Build history of the part. All positions in model axes, mm. A direction names the side the tool comes from. Give positions to 0.01 mm unless a question says otherwise; leave off trailing zeros. Write each loop counter-clockwise with the first axis right and the second up, starting at its lowest first coordinate (ties: lowest second). Pieces come first, ordered by that corner, then holes. Notation, with made-up numbers: M -13,36 L 33,36 A7 cw 33,40 Z; hole C 2,86.25 d11. An arc over 180 degrees is marked long. One line per item, written item: value. Start each with the question number.
from build123d import *

# Parameters (mm, degrees)
SKETCH1_W           = 254
SKETCH1_H           = 46.99
BOSS_EXTRUDE1_DEPTH = 3.0988
FILLET1_R           = 6.35
SKETCH2_W           = 63.5
SKETCH2_H           = 5.715
CUT_EXTRUDE1_DEPTH  = 130.192173085
SKETCH3_W           = 38.1
SKETCH3_H           = 5.08
CUT_EXTRUDE2_DEPTH  = 130.192173085
CUT_EXTRUDE3_DEPTH  = 130.192173085
FILLET2_R           = 6.35


with BuildPart() as part:
    # Sketch1 → Boss-Extrude1 (new body)
    with BuildSketch(Plane.XY):
        Rectangle(SKETCH1_W, SKETCH1_H)
    extrude(amount=BOSS_EXTRUDE1_DEPTH)

    # Fillet1
    fillet1_edges = [part.edges().sort_by_distance(p)[0] for p in [
        (-127, 23.495, 1.5494),
        (127, 23.495, 1.5494),
    ]]
    fillet(fillet1_edges, radius=FILLET1_R)

    # Sketch2 → Cut-Extrude1 (cut, through all)
    with BuildSketch(Plane.XY.offset(3.0988)):
        with Locations((-95.25, -20.6375)):
            Rectangle(SKETCH2_W, SKETCH2_H)
        with Locations((95.25, -20.6375)):
            Rectangle(SKETCH2_W, SKETCH2_H)
    extrude(amount=-CUT_EXTRUDE1_DEPTH, mode=Mode.SUBTRACT)

    # Sketch3 → Cut-Extrude2 (cut, through all)
    with BuildSketch(Plane.XY.offset(3.0988)):
        with Locations((-102.87, -15.24)):
            Rectangle(SKETCH3_W, SKETCH3_H)
        with Locations((102.87, -15.24)):
            Rectangle(SKETCH3_W, SKETCH3_H)
    extrude(amount=-CUT_EXTRUDE2_DEPTH, mode=Mode.SUBTRACT)

    # Sketch4 → Cut-Extrude3 (cut, through all)
    with BuildSketch(Plane.XY.offset(3.0988)):
        Polygon((-77.47, -6.35), (77.47, -6.35), (120.65, -6.35), (120.65, 17.145), (-120.65, 17.145), (-120.65, -6.35), align=None)
    extrude(amount=-CUT_EXTRUDE3_DEPTH, mode=Mode.SUBTRACT)

    # Fillet2
    fillet2_edges = [part.edges().sort_by_distance(p)[0] for p in [
        (-120.65, 17.145, 1.5494),
        (120.65, 17.145, 1.5494),
        (120.65, -6.35, 1.5494),
        (-120.65, -6.35, 1.5494),
    ]]
    fillet(fillet2_edges, radius=FILLET2_R)


solid = part.part
1) Band-saw the part on B-B (z = 2.4). List the corners of the cut face in (x, y) (3 decimals).
2) Tool access for faces 1 (the face through (118.839, 15.235, 1.528)), 2 (the face through (-125.189, 21.585, 1.571)): list every direction of +Z, -Z, +X, -X, +Y, -Y with a clear straight run to the whole face (end or side of a thin tool).
3) Band-saw the part on D-D (y = -20). List the corners of the cut face in (x, z), then the cut area to 3 significant figures.
4) Probe line 1 along Y through (x, z) = (-3, 0.6) (3 decimals); line 2 along Y through (x, z) = (-112, 0.2) (3 decimals); line 3 along X through (y, z) = (0.5, 2.9). List the from-to ranges inside material, lowest first. Write a range as from..to.
5) Band-saw the part on A-A (x = 100). List the corners of the cut face in (y, z) (3 decimals).
6) Mould opens along Y. For faces 3 (the face through (125.189, 21.585, 1.571)), 4 (the face through (-118.84, -4.44, 1.53)), 5 (the face through (118.84, -4.44, 1.53)), 6 (the face through (-10, -7, 0)) say: released by +Y, released by -Y, zero draft, split by the parting line, or undercut.
7) Band-saw the part on C-C (x = -70). List the corners of the cut face in (y, z) (3 decimals).
8) Drop flat-ended pins along their axis: P1, Ø0.9, axis at x = 95, z = 1.5, coming from the -Y side; P2, Ø0.9, axis at x = -72, z = 2, coming from the -Y side; P3, Ø1.5, axis at y = -21.5, z = 2, coming from the +X side. Give the stop position or say it passes through.
Model answer:
1. outline: M -127,-17.78 L -121.92,-17.78 L -121.92,-12.7 L -83.82,-12.7 L -83.82,-17.78 L -63.5,-17.78 L -63.5,-23.495 L 63.5,-23.495 L 63.5,-17.78 L 83.82,-17.78 L 83.82,-12.7 L 121.92,-12.7 L 121.92,-17.78 L 127,-17.78 L 127,17.145 A6.35 ccw 120.65,23.495 L -120.65,23.495 A6.35 ccw -127,17.145 Z; hole M -120.65,0 A6.35 ccw -114.3,-6.35 L 114.3,-6.35 A6.35 ccw 120.65,0 L 120.65,10.795 A6.35 ccw 114.3,17.145 L -114.3,17.145 A6.35 ccw -120.65,10.795 Z
2. face 1: +Z, -Z
2. face 2: +Z, -Z, -X, +Y
3. outline: M -63.5,0 L 63.5,0 L 63.5,3.1 L -63.5,3.1 Z
3. area: 394 mm²
4. line 1: y = -23.495..-6.35, 17.145..23.495
4. line 2: y = -12.7..-6.35, 17.145..23.495
4. line 3: x = -127..-120.65, 120.65..127
5. outline: M -12.7,0 L -6.35,0 L -6.35,3.099 L -12.7,3.099 Z; M 17.145,0 L 23.495,0 L 23.495,3.099 L 17.145,3.099 Z
6. face 3: released by +Y
6. face 4: undercut
6. face 5: undercut
6. face 6: zero draft
7. outline: M -17.78,0 L -6.35,0 L -6.35,3.099 L -17.78,3.099 Z; M 17.145,0 L 23.495,0 L 23.495,3.099 L 17.145,3.099 Z
8. P1: stops at y = -12.7
8. P2: stops at y = -17.78
8. P3: stops at x = 63.5
